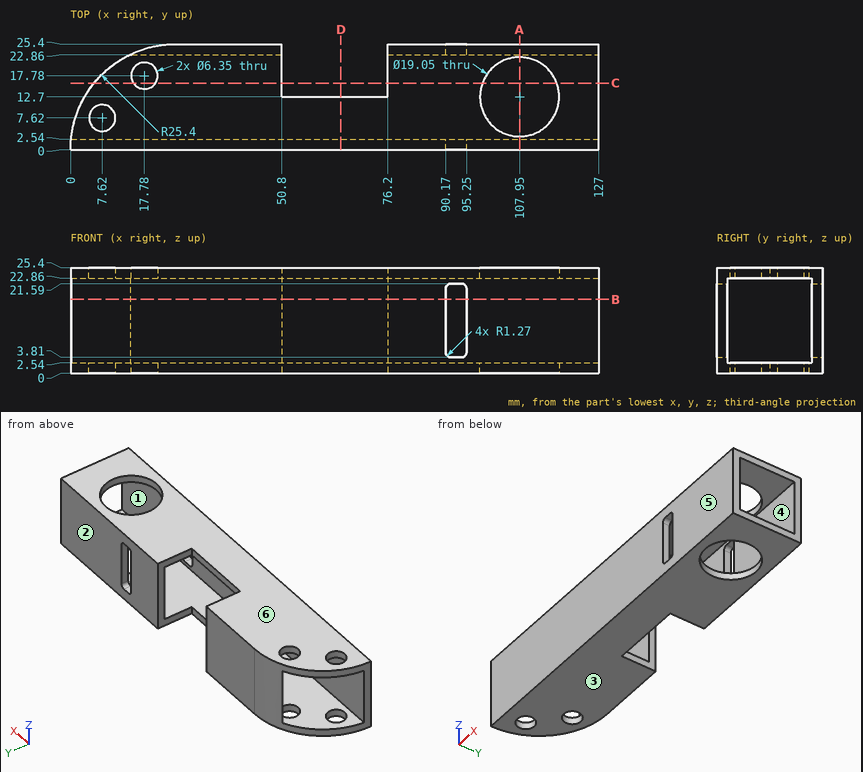
Answer from the drawing. Dimensions are ordinates in mm from the lowest x, y and z of the part. A direction names the side the tool comes from. Round coordinates to 2 decimals unless told otherwise and drop trailing zeros. Loops run counter-clockwise (first coordinate to the right, second up) from the corner with the lowest first, then second, coordinate; pieces in that order, holes last. Notation, with made-up numbers: (71.5, -3) - (80.5, -3) arc R37 cw to (80.5, 33) - close; hole circle Ø7 at (-1.5, 16.5). An arc over 180 degrees is marked (long way). Return JSON: item names as keys, results as strings. Group by question number.
1. The part is cut by section D-D on x = 65. Determine the outline of the cut face in (y, z).
2. The part is cut by section C-C on y = 16. State how many separate pieces and enclosed holes the cut face has, then the cut area to 3 significant figures.
3. Which of the six approach directions +Z, -Z, +X, -X, +Y, -Y give full straight-line access (tool end or side, diameter ignored) to the marked faces 1 and 2?
4. Each of these flat-tipped pins is pushed along its axis until it touches: P1, Ø8.5, axis at x = 17.78, y = 17.78, coming from the -Z side; P2, Ø11.5, axis at x = 107.95, y = 12.7, coming from the -Z side; P3, Ø3, axis at x = 66, z = 23.5, coming from the +Y side; P4, Ø12, axis at y = 10, z = 22.5, coming from the -X side. Where does it stop, or does it pass through?
5. The mould has two halves that part along Z. Classify the marked faces 3, 4, 5 and 6: pulls with the +Z half, pulls with the -Z half, needs draft (parallel to the pull), parting line crosses it, or undercut.
6. The part is cut by section B-B on z = 17.75. Determine the outline of the cut face in (x, y).
7. Consider probe 1 along Y at (x, z) = (50, 10.5); probe 2 along Y at (x, z) = (107.95, 1.15) (3 decimals). Determine where each line is inside the solid, lowest interval first.
8. The part is cut by section A-A on x = 107.95. Determine the outline of the cut face in (y, z) (3 decimals).
Resolved:
{
 "1": {"outline": "(0, 0) - (12.7, 0) - (12.7, 2.54) - (2.54, 2.54) - (2.54, 22.86) - (12.7, 22.86) - (12.7, 25.4) - (0, 25.4) - close"},
 "2": {"separate pieces": "8", "enclosed holes": "0", "area": "370 mm²"},
 "3": {"face 1": "+X, -X", "face 2": "+Z, -Z, +X, -X, +Y"},
 "4": {"P1": "stops at z = 0", "P2": "passes through", "P3": "stops at y = 12.7", "P4": "stops at x = 0.32"},
 "5": {"face 3": "pulls with the -Z half", "face 4": "undercut", "face 5": "needs draft", "face 6": "pulls with the +Z half"},
 "6": {"outline": "(0, 0) - (90.17, 0) - (90.17, 2.54) - (0.13, 2.54) arc R25.4 ccw to start; (14.33, 22.86) - (50.8, 22.86) - (50.8, 25.4) - (25.4, 25.4) arc R25.4 ccw to start; (76.2, 22.86) - (90.17, 22.86) - (90.17, 25.4) - (76.2, 25.4) - close; (95.25, 0) - (127, 0) - (127, 2.54) - (95.25, 2.54) - close; (95.25, 22.86) - (127, 22.86) - (127, 25.4) - (95.25, 25.4) - close"},
 "7": {"probe 1": "y = 0 to 2.54, 22.86 to 25.4", "probe 2": "y = 0 to 3.175, 22.225 to 25.4"},
 "8": {"outline": "(0, 0) - (3.175, 0) - (3.175, 2.54) - (2.54, 2.54) - (2.54, 22.86) - (3.175, 22.86) - (3.175, 25.4) - (0, 25.4) - close; (22.225, 0) - (25.4, 0) - (25.4, 25.4) - (22.225, 25.4) - (22.225, 22.86) - (22.86, 22.86) - (22.86, 2.54) - (22.225, 2.54) - close"}
}
